Here's the drawing with two shaded views (mm, measured from the low corner). I have some questions. Round coordinates to 2 decimals unless told otherwise and drop trailing zeros. Order: outer loops, then holes, each group sorted by start corner. A loop starts at its lowest first (then second) coordinate and runs counter-clockwise, first axis right, second up. Notation, with made-up numbers: (62, -13) - (120, -13) arc R29 cw to (120, 11) - close; hole circle Ø10 at (34, -12.75). An arc over 180 degrees is marked (long way). One line per item, written item: value.
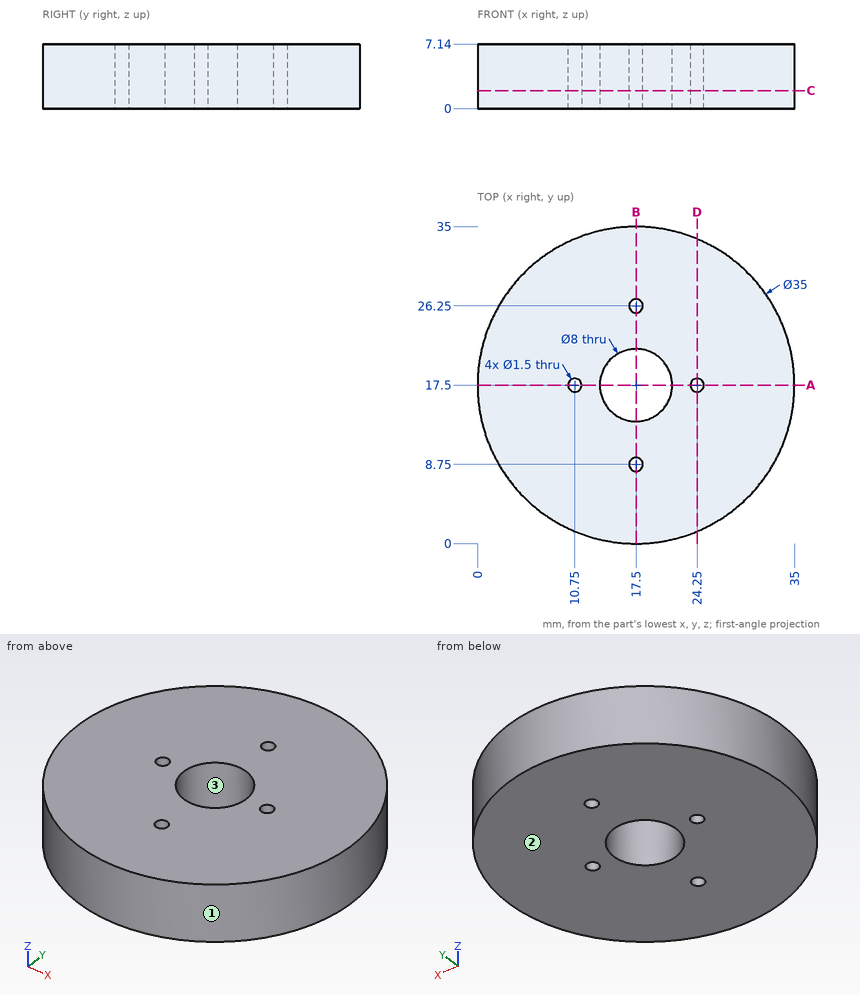
Q1. We'd pull the mould along X, two halves only. Please class the marked faces 1, 2 and 3: released by +X, released by -X, zero draft, split by the parting line, or undercut.
Results list:
face 1: split by the parting line
face 2: zero draft
face 3: undercut
Q2. If I drill on line 1 along Y through (x, z) = (17.5, 3.25); line 2 along Y through (x, z) = (18, 1.75); line 3 along X through (y, z) = (8.75, 3), over which ranges is the centre line in solid material (lowest first)?
Results list:
line 1: 0 to 8, 9.5 to 13.5, 21.5 to 25.5, 27 to 35
line 2: 0.01 to 8.19, 9.31 to 13.53, 21.47 to 25.69, 26.81 to 34.99
line 3: 2.34 to 16.75, 18.25 to 32.66
Q3. If we section it at D-D, the plane x = 24.25: Please give me the cut outline in (y, z).
Results list:
outline: (1.35, 0) - (16.75, 0) - (16.75, 7.14) - (1.35, 7.14) - close; (18.25, 0) - (33.65, 0) - (33.65, 7.14) - (18.25, 7.14) - close
Q4. Will these pins go through, and if not, where does the flat tip stop? pin 1 (1.5 mm diameter, centred on y = 4, z = 5.5, fed in from +X); pin 2 (3 mm diameter, centred on y = 20.5, z = 5, fed in from -X).
Results list:
pin 1: x = 29.49
pin 2: x = 0.06
Q5. If we section it at A-A, the plane y = 17.5: Please give me the cut outline in (x, z), then the cut area to 3 significant figures.
Results list:
outline: (0, 0) - (10, 0) - (10, 7.14) - (0, 7.14) - close; (11.5, 0) - (13.5, 0) - (13.5, 7.14) - (11.5, 7.14) - close; (21.5, 0) - (23.5, 0) - (23.5, 7.14) - (21.5, 7.14) - close; (25, 0) - (35, 0) - (35, 7.14) - (25, 7.14) - close
area: 171 mm²
Q6. If we section it at B-B, the plane x = 17.5: Please give me the cut outline in (y, z), then the cut area to 3 significant figures.
Results list:
outline: (0, 0) - (8, 0) - (8, 7.14) - (0, 7.14) - close; (9.5, 0) - (13.5, 0) - (13.5, 7.14) - (9.5, 7.14) - close; (21.5, 0) - (25.5, 0) - (25.5, 7.14) - (21.5, 7.14) - close; (27, 0) - (35, 0) - (35, 7.14) - (27, 7.14) - close
area: 171 mm²
Q7. If we section it at C-C, the plane z = 2: Please give me the cut outline in (x, y), then the cut area to 3 significant figures.
Results list:
outline: circle Ø35 at (17.5, 17.5); hole circle Ø1.5 at (10.75, 17.5); hole circle Ø8 at (17.5, 17.5); hole circle Ø1.5 at (17.5, 8.75); hole circle Ø1.5 at (17.5, 26.25); hole circle Ø1.5 at (24.25, 17.5)
area: 905 mm²
